For this review, take the finished solid that the model builds, in its own axes (mm). A direction names the side the tool comes from. Coordinates: 2 decimals unless noted, no trailing zeros. Order: outer loops, then holes, each group sorted by start corner. A loop starts at its lowest first (then second) coordinate and runs counter-clockwise, first axis right, second up. Notation, with made-up numbers: (41, 3.25) -> (98, 3.25) arc R29 ccw to (98, 27.25) -> close; hole circle Ø10 at (1, 8). An arc over 180 degrees is marked (long way). Return JSON: item names as keys, results as strings. Group by question number.
Item 1: Draft analysis for pull direction X (two halves, no side actions). For faces 5 (the flat face through (343, 19.5, 0)), 6 (the flat face through (-38.708, 14.1, -22.1)), 7 (the flat face through (271.292, -29, 2)), 8 (the flat face through (78, 21.5, 0)), state which applies: +X half, -X half, draft (parallel to the pull), parting line (faces both ways), or undercut.
Item 2: For line 1 along X through (y, z) = (-10, -29); line 2 along Z through (x, y) = (-38.5, -3); line 3 along Z through (x, y) = (268, 6), list the stretches that pass through material, from the lowest coordinate up.
Item 3: Take a section at A-A (x = 148). Write out the cut boundary in (y, z).
Item 4: Machinability: for faces 1 (the cylindrical face through (347.88, 23.846, -7.509)), 2 (the cylindrical face through (196.35, 31, -9.76)), 3 (the cylindrical face through (113.326, 24.542, -0.176)), 4 (the cylindrical face through (-75.944, 23.846, -7.509)), which of the approach directions +Z, -Z, +X, -X, +Y, -Y give a long, thin tool a straight path to every point of the face, cutting with its end or side? Answer none if there is none.
Item 5: Take a section at B-B (x = -23). Write out the cut boundary in (y, z), then the cut area to 3 significant figures.
Item 6: Insertion check: pin 1 (1.5 mm diameter, centred on x = 325, z = -0.5, fed in from -Y); pin 2 (5.5 mm diameter, centred on x = 68, y = 24, fed in from -Z); pin 3 (5 mm diameter, centred on x = 344, y = 21.5, fed in from -Z); pin 4 (5 mm diameter, centred on y = 24, z = 9, fed in from -X). Each pin has a flat end and moves straight along its axis. Give the tip position at first contact, or say it passes through.
```python
from build123d import *

# Parameters (mm, degrees)
CHAMFER1_SIZE      = 0.5
FILLET1_R          = 1
CUT_EXTRUDE1_DEPTH = 6
CUT_EXTRUDE2_DEPTH = 5.5


with BuildPart() as part:
    # Sketch1 → Revolve1 (revolve)
    with BuildSketch(Plane.XY):
        Polygon((-113.708057171, 0), (-113.708057171, 25), (-38.708057171, 25), (-38.708057171, 27.5), (119.291942829, 27.5), (119.291942829, 32.5), (271.291942829, 32.5), (271.291942829, 27.5), (304.291942829, 27.5), (304.291942829, 25), (389.291942829, 25), (389.291942829, 0), (178.819444444, 0), align=None)
    revolve(axis=Axis((178.819444444, 0, 0), (-1, 0, 0)))

    # Chamfer1
    chamfer1_edges = [part.edges().sort_by_distance(p)[0] for p in [
        (304.291942829, -27.5, 0),
        (271.291942829, -32.5, 0),
        (119.291942829, -32.5, 0),
        (-38.708057171, -27.5, 0),
        (-113.708057171, -25, 0),
    ]]
    chamfer(chamfer1_edges, length=CHAMFER1_SIZE)

    # Fillet1
    fillet1_edges = [part.edges().sort_by_distance(p)[0] for p in [
        (304.291942829, -25, 0),
        (271.291942829, -27.5, 0),
        (119.291942829, -27.5, 0),
        (-38.708057171, -25, 0),
    ]]
    fillet(fillet1_edges, radius=FILLET1_R)

    # Sketch3 → Cut-Extrude1 (cut)
    with BuildSketch(Plane(origin=(0, 27.5, 0), x_dir=(1, 0, 0), z_dir=(0, 1, 0))):
        with BuildLine():
            Line((50.328098338, 8), (105.328098338, 8))
            ThreePointArc((105.328098338, 8), (113.328098338, 0), (105.328098338, -8))
            Line((105.328098338, -8), (50.328098338, -8))
            ThreePointArc((50.328098338, -8), (42.328098338, 0), (50.328098338, 8))
        make_face()
    extrude(amount=-CUT_EXTRUDE1_DEPTH, mode=Mode.SUBTRACT)

    # Sketch4 → Cut-Extrude2 (cut)
    with BuildSketch(Plane(origin=(0, 25, 0), x_dir=(1, 0, 0), z_dir=(0, 1, 0))):
        with BuildLine():
            Line((317.435334748, 7), (367.435334748, 7))
            ThreePointArc((367.435334748, 7), (374.435334748, 0), (367.435334748, -7))
            Line((367.435334748, -7), (317.435334748, -7))
            ThreePointArc((317.435334748, -7), (310.435334748, 0), (317.435334748, 7))
        make_face()
    extrude(amount=-CUT_EXTRUDE2_DEPTH, mode=Mode.SUBTRACT)


solid = part.part
```
Findings below:
{
 "1": {"face 5": "undercut", "face 6": "-X half", "face 7": "+X half", "face 8": "undercut"},
 "2": {"line 1": "x = 119.29 to 271.29", "line 2": "z = -27.04 to 27.04", "line 3": "z = -31.94 to 31.94"},
 "3": {"outline": "circle Ø65 at (0, 0)"},
 "4": {"face 1": "+X", "face 2": "+X, -X", "face 3": "+Y", "face 4": "-X"},
 "5": {"outline": "circle Ø55 at (0, 0)", "area": "2,380 mm2"},
 "6": {"pin 1": "stops at y = -25", "pin 2": "stops at z = -17.46", "pin 3": "stops at z = -16.25", "pin 4": "stops at x = -113.71"}
}
